Autodesk Inventor part; units mm, degrees
ref_plane "YZ Plane" through (0, 0, 0) normal (1, 0, 0) x (0, 1, 0)
ref_plane "XZ Plane" through (0, 0, 0) normal (0, 1, 0) x (-1, 0, 0)
ref_plane "XY Plane" through (0, 0, 0) normal (0, 0, 1) x (1, 0, 0)
sketch "Эскиз1" plane through (0, 0, 0) normal (0, 0, 1) x (1, 0, 0)
  circle A0 centre (60.6218, 35) radius 7.5
  circle A1 centre (60.6218, 35) radius 7
  point P0 (0, 0)
  dimension "d0" = 14
extrude "Выдавливание1" add sketch "Эскиз1" along normal blind 29.5 contours A1
sketch "Эскиз2" plane through (60.6218, 35, 29.5) normal (0, 0, 1) x (1, 0, 0)
  line L0 (12.5, 11.1132) -> (-12.5, 11.1132)
  line L1 (-12.5, 11.1132) -> (-12.5, -11.1132)
  line L2 (-12.5, -11.1132) -> (12.5, -11.1132)
  line L3 (12.5, -11.1132) -> (12.5, 11.1132)
  line L4 (12.5, 11.1132) -> (-12.5, -11.1132) construction
  line L5 (-12.5, 11.1132) -> (12.5, -11.1132) construction
  point P0 (-60.6218, -35)
  point P1 (0, 0)
  dimension "d3" = 25
extrude "Выдавливание2" add sketch "Эскиз2" along normal blind 40
sketch "Эскиз3" plane through (60.6218, 35, 69.5) normal (0, 0, 1) x (1, 0, 0)
  circle A0 centre (0, 0) radius 7.5
  point P0 (-60.6218, -35)
  dimension "d6" = 15
extrude "Выдавливание3" cut sketch "Эскиз3" against normal blind 34.25
properties part number "Гайка"
Source: CAD feature listing. Evaluate the final solid. Frame: model axes, mm. A direction names the side the tool comes from. Give positions to 0.01 mm unless a question says otherwise; leave off trailing zeros. Write each loop counter-clockwise with the first axis right and the second up, starting at its lowest first coordinate (ties: lowest second). Pieces come first, ordered by that corner, then holes. Notation, with made-up numbers: (-5, 81) -> (31, 81) arc R17 cw to (31, 107) -> close; hole circle Ø4 at (69.25, -18). An arc over 180 degrees is marked (long way). Write item = value, one per line.
Q1. Line query: line 1 (Z direction, x = 59, y = 30.25); line 2 (Z direction, x = 52.5, y = 30.25); line 3 (Y direction, x = 61.25, z = 43.5). Output: solid intervals per line, ascending. Write a range as from..to.
Here are the results:
line_1 = 0..35.25
line_2 = 29.5..69.5
line_3 = 23.89..27.53, 42.47..46.11
Q2. First-contact query: pin 1 (2 mm diameter, centred on x = 58, z = 25, fed in from +Y); pin 2 (3 mm diameter, centred on y = 35, z = 9.5, fed in from +X); pin 3 (10 mm diameter, centred on x = 69.5, z = 18, fed in from +Y). Flat tips, straight axial feed; report the tip coordinate or a pass-through.
Here are the results:
pin_1 = 41.81
pin_2 = 67.62
pin_3 = 40.83
Q3. Mould query, pull axis X, two halves, no side actions, for faces 1 (the face through (60, 23.887, 49)), 2 (the face through (73.122, 35, 49)), 3 (the face through (61, 35, 35.25)). Classes: +X half, -X half, draft (parallel to the pull), parting line (faces both ways), or undercut.
Here are the results:
face_1 = draft
face_2 = +X half
face_3 = undercut
Q4. Cut plane B-B on y = 35. Return loops of the section in (x, z), then the cut area to 3 significant figures.
Here are the results:
outline = (48.12, 29.5) -> (53.62, 29.5) -> (53.62, 0) -> (67.62, 0) -> (67.62, 29.5) -> (73.12, 29.5) -> (73.12, 69.5) -> (68.12, 69.5) -> (68.12, 35.25) -> (53.12, 35.25) -> (53.12, 69.5) -> (48.12, 69.5) -> close
area = 899 mm²
Q5. Reachability of faces 4 (the face through (58.996, 27.678, 52.615)), 5 (the face through (60, 43, 69.5)), 6 (the face through (60, 43, 29.5)) from +Z, -Z, +X, -X, +Y, -Y: full face, straight path, thin tool, end or side. Return the list, or none.
Here are the results:
face_4 = +Z
face_5 = +Z, +X, -X, +Y, -Y
face_6 = -Z
Q6. Cut plane D-D on z = 19. Return loops of the section in (x, y), then the cut area to 3 significant figures.
Here are the results:
outline = circle Ø14 at (60.62, 35)
area = 154 mm²
Q7. Cut plane A-A on z = 46. Return loops of the section in (x, y), then the cut area to 3 significant figures.
Here are the results:
outline = (48.12, 23.89) -> (73.12, 23.89) -> (73.12, 46.11) -> (48.12, 46.11) -> close; hole circle Ø15 at (60.62, 35)
area = 379 mm²
Q8. Cut plane C-C on x = 54.75. Return loops of the section in (y, z), then the cut area to 3 significant figures.
Here are the results:
outline = (23.89, 29.5) -> (31.19, 29.5) -> (31.19, 0) -> (38.81, 0) -> (38.81, 29.5) -> (46.11, 29.5) -> (46.11, 69.5) -> (39.67, 69.5) -> (39.67, 35.25) -> (30.33, 35.25) -> (30.33, 69.5) -> (23.89, 69.5) -> close
area = 794 mm²
